Autodesk Inventor part; units mm, degrees
ref_plane "YZ Plane" through (0, 0, 0) normal (1, 0, 0) x (0, 1, 0)
ref_plane "XZ Plane" through (0, 0, 0) normal (0, 1, 0) x (-1, 0, 0)
ref_plane "XY Plane" through (0, 0, 0) normal (0, 0, 1) x (1, 0, 0)
sketch "Sketch1" plane through (0, 0, 0) normal (0, 0, 1) x (1, 0, 0)
  line L0 (0, 0) -> (308, 0)
  line L1 (308, 0) -> (308, 270)
  line L2 (308, 270) -> (0, 270)
  line L3 (0, 270) -> (0, 0)
  dimension "d0" = 308
  dimension "d1" = 270
extrude "Extrusion1" add sketch "Sketch1" along normal blind 20
sketch "Sketch2" plane through (0, 0, 20) normal (0, 0, 1) x (1, 0, 0)
  line L0 (150.8623, 77.3843) -> (180.284, 77.3843)
  line L1 (180.284, 77.3843) -> (214.6934, 126.131)
  line L2 (214.6934, 126.131) -> (197.4887, 161.9741)
  line L3 (197.4887, 161.9741) -> (180.284, 217.8894)
  line L4 (180.284, 217.8894) -> (163.9156, 161.9741)
  line L5 (163.9156, 161.9741) -> (150.8623, 161.9741)
  line L6 (150.8623, 161.9741) -> (150.8623, 77.3843) construction
  line L7 (150.8623, 77.3843) -> (121.4405, 77.3843)
  line L8 (121.4405, 77.3843) -> (87.0311, 126.131)
  line L9 (87.0311, 126.131) -> (104.2358, 161.9741)
  line L10 (104.2358, 161.9741) -> (121.4405, 217.8894)
  line L11 (121.4405, 217.8894) -> (137.8089, 161.9741)
  line L12 (137.8089, 161.9741) -> (150.8623, 161.9741)
  line L13 (308, 0) -> (308, 270)
  line L14 (144.5227, 131.6434) -> (112.8382, 144.3477)
  line L15 (112.8382, 144.3477) -> (112.8382, 131.6434)
  line L16 (112.8382, 131.6434) -> (144.5227, 131.6434)
  line L17 (157.2018, 131.6434) -> (188.8863, 144.3477)
  line L18 (188.8863, 144.3477) -> (188.8863, 131.6434)
  line L19 (188.8863, 131.6434) -> (157.2018, 131.6434)
  line L20 (150.8623, 117.5428) -> (137.8089, 101.7577)
  line L21 (137.8089, 101.7577) -> (163.9156, 101.7577)
  line L22 (163.9156, 101.7577) -> (150.8623, 117.5428)
  line L23 (212.9598, 126.2762) -> (179.5067, 78.8843)
  line L24 (179.5067, 78.8843) -> (150.8623, 78.8843)
  line L25 (150.8623, 78.8843) -> (122.2178, 78.8843)
  line L26 (122.2178, 78.8843) -> (88.7647, 126.2762)
  line L27 (88.7647, 126.2762) -> (105.6366, 161.426)
  line L28 (105.6366, 161.426) -> (121.4047, 212.6725)
  line L29 (121.4047, 212.6725) -> (136.6851, 160.4741)
  line L30 (136.6851, 160.4741) -> (150.8623, 160.4741)
  line L31 (150.8623, 160.4741) -> (165.0395, 160.4741)
  line L32 (165.0395, 160.4741) -> (180.3198, 212.6725)
  line L33 (180.3198, 212.6725) -> (196.0879, 161.426)
  line L34 (196.0879, 161.426) -> (212.9598, 126.2762)
  line L35 (111.3382, 146.5653) -> (150.8623, 130.7176)
  line L36 (152.2942, 130.1434) -> (111.3382, 130.1434)
  line L37 (111.3382, 130.1434) -> (111.3382, 146.5653)
  line L38 (150.8623, 130.7176) -> (190.3863, 146.5653)
  line L39 (190.3863, 146.5653) -> (190.3863, 130.1434)
  line L40 (190.3863, 130.1434) -> (149.4303, 130.1434)
  line L41 (150.8623, 119.8965) -> (134.6221, 100.2577)
  line L42 (134.6221, 100.2577) -> (167.1025, 100.2577)
  line L43 (167.1025, 100.2577) -> (150.8623, 119.8965)
  line L44 (74.5244, 66.3096) -> (229.3713, 66.3096) construction
  line L45 (229.3713, 66.3096) -> (229.3713, 36.329) construction
  line L46 (229.3713, 36.329) -> (74.5244, 36.329) construction
  line L47 (74.5244, 36.329) -> (74.5244, 66.3096) construction
  line L48 (208.446, 49.8524) -> (208.446, 52.8954)
  line L49 (97.2006, 52.8954) -> (97.2006, 49.8524)
  spline S0 degree 2 poles (98.2109, 52.4396) (98.2109, 45.1875) (95.3431, 41.5752) knots 0 0 0 1 1 1
  spline S1 degree 2 poles (95.3431, 41.5752) (92.9717, 38.5145) (88.0359, 37.5494) knots 0 0 0 1 1 1
  spline S2 degree 2 poles (88.0359, 37.5494) (85.0303, 36.9703) (78.0264, 36.9703) knots 0 0 0 1 1 1
  line L50 (78.0264, 36.9703) -> (78.0264, 66.3096)
  spline S3 degree 2 poles (78.0264, 66.3096) (88.4219, 66.3096) (92.1169, 64.5724) knots 0 0 0 1 1 1
  spline S4 degree 2 poles (92.1169, 64.5724) (98.2109, 61.7598) (98.2109, 52.4396) knots 0 0 0 1 1 1
  spline S5 degree 2 poles (96.0877, 52.4396) (96.0877, 60.2707) (91.0139, 62.78) knots 0 0 0 1 1 1
  spline S6 degree 2 poles (91.0139, 62.78) (88.0359, 64.1863) (80.1496, 64.1863) knots 0 0 0 1 1 1
  line L51 (80.1496, 64.1863) -> (80.1496, 39.0935)
  spline S7 degree 2 poles (80.1496, 39.0935) (87.9808, 39.0935) (91.0139, 40.7756) knots 0 0 0 1 1 1
  spline S8 degree 2 poles (91.0139, 40.7756) (96.0877, 43.5882) (96.0877, 52.4396) knots 0 0 0 1 1 1
  spline S9 degree 2 poles (227.425, 41.0513) (225.219, 38.4042) (221.0277, 36.3912) (218.1599, 36.3912) knots 0 0 0 1 2 2 2
  spline S10 degree 2 poles (218.1599, 36.3912) (213.4998, 36.3912) (207.5713, 44.7463) (207.5713, 51.6951) knots 0 0 0 1 2 2 2
  spline S11 degree 2 poles (207.5713, 51.6951) (207.5713, 59.2781) (211.1284, 63.1385) knots 0 0 0 1 1 1
  spline S12 degree 2 poles (211.1284, 63.1385) (214.0238, 66.3096) (218.1599, 66.3096) knots 0 0 0 1 1 1
  spline S13 degree 2 poles (218.1599, 66.3096) (221.331, 66.3096) (225.219, 64.1863) (226.6804, 61.5392) knots 0 0 0 1 2 2 2
  spline S14 degree 2 poles (226.6804, 61.5392) (226.8459, 61.291) (226.8459, 61.0153) knots 0 0 0 1 1 1
  spline S15 degree 2 poles (226.8459, 61.0153) (226.8459, 59.9674) (225.7429, 59.9674) knots 0 0 0 1 1 1
  spline S16 degree 2 poles (225.7429, 59.9674) (225.219, 59.9674) (224.8881, 60.4913) knots 0 0 0 1 1 1
  spline S17 degree 2 poles (224.8881, 60.4913) (222.7649, 64.1863) (218.2702, 64.1863) knots 0 0 0 1 1 1
  spline S18 degree 2 poles (218.2702, 64.1863) (214.8786, 64.1863) (212.5623, 61.4289) knots 0 0 0 1 1 1
  spline S19 degree 2 poles (212.5623, 61.4289) (209.6946, 58.0372) (209.6946, 51.6951) knots 0 0 0 1 1 1
  spline S20 degree 2 poles (209.6946, 51.6951) (209.6946, 45.932) (214.6855, 38.5145) (218.2702, 38.5145) knots 0 0 0 1 2 2 2
  spline S21 degree 2 poles (218.2702, 38.5145) (222.6821, 38.5145) (225.7429, 42.43) knots 0 0 0 1 1 1
  spline S22 degree 2 poles (225.7429, 42.43) (226.0462, 42.8437) (226.5977, 42.8437) knots 0 0 0 1 1 1
  spline S23 degree 2 poles (226.5977, 42.8437) (227.7007, 42.8437) (227.7007, 41.7407) knots 0 0 0 1 1 1
  spline S24 degree 2 poles (227.7007, 41.7407) (227.7007, 41.3546) (227.425, 41.0513) knots 0 0 0 1 1 1
  point P0 (0, 0)
  point P1 (150.8623, 130.1434)
  dimension "d5" = 1.5
  dimension "d6" = 1.5
  dimension "d7" = 1.5
  dimension "d8" = 1.5
extrude "Extrusion2" cut sketch "Sketch2" against normal blind 8
properties part number "Tablero_DC_007"
The listing builds one solid part. Answer for the finished solid, in the listing's coordinates (mm). A direction names the side the tool comes from. Coordinates: 2 decimals unless noted, no trailing zeros.
Q1. Which of the six approach directions +Z, -Z, +X, -X, +Y, -Y give full straight-line access (tool end or side, diameter ignored) to faces 3 (the face through (172.822, 137.907, 16.056)), 4 (the face through (152, 167, 20))?
Q2. A cutting plane is placed at A-A, the plane z = 16.5. State how many separate pieces and enclosed holes the cut face has, and give its area (3 significant figures).
Q3. For a pull along X with two mould halves and no side action, classify faces 1 (the face through (151, 108, 20)), 2 (the face through (173, 131.643, 16)) as pulls with the +X half, pulls with the -X half, needs draft (parallel to the pull), parting line crosses it, or undercut.
Q4. Consider line 1 (X direction, y = 157.5, z = 13.25); line 2 (X direction, y = 202.5, z = 14.75); line 3 (Y direction, x = 99.5, z = 12.25). Determine where each line is inside the solid, lowest interval first.
Q5. Given P1, Ø4, axis at y = 224.5, z = 11.5, coming from the -X side, flat-ended and moving along its own axis, determine where the tip first touches the part or whether it passes through.
Answers follow:
1. face 3: +Z
1. face 4: +Z, +X, -X, +Y, -Y
2. separate pieces: 6
2. enclosed holes: 5
2. area: 81,700 mm2
3. face 1: needs draft
3. face 2: undercut
4. line 1: x = 0 to 102.09, 103.75 to 197.97, 199.64 to 308
4. line 2: x = 0 to 116.71, 118.27 to 124.38, 125.95 to 175.78, 177.34 to 183.45, 185.02 to 308
4. line 3: y = 0 to 108.47, 111.07 to 148.64, 152.11 to 270
5. P1: stops at x = 0
